Work out the finished part from the listing and answer in its coordinate system (mm). Face numbers are marked on the shaded views. A direction names the side the tool comes from. Round coordinates to 2 decimals unless told otherwise and drop trailing zeros. Order: outer loops, then holes, each group sorted by start corner. A loop starts at its lowest first (then second) coordinate and runs counter-clockwise, first axis right, second up. Notation, with made-up numbers: (35.25, 75.5) - (55.25, 75.5) arc R28 ccw to (55.25, 110.5) - close; hole circle Ø8 at (65.5, -1.75). An arc over 180 degrees is marked (long way). Put each result on its own line as item: value.
Autodesk Inventor part; units mm, degrees
ref_plane "YZ Plane" through (0, 0, 0) normal (1, 0, 0) x (0, 1, 0)
ref_plane "XZ Plane" through (0, 0, 0) normal (0, 1, 0) x (-1, 0, 0)
ref_plane "XY Plane" through (0, 0, 0) normal (0, 0, 1) x (1, 0, 0)
sketch "Sketch1" plane through (0, 0, 0) normal (1, 0, 0) x (0, 1, 0)
  line L0 (0, 0) -> (7.62, 0)
  line L1 (7.62, 0) -> (7.62, -15.24)
  line L2 (7.62, -15.24) -> (0, -15.24)
  line L3 (0, -15.24) -> (0, 0)
  dimension "d0" = 7.62
  dimension "d1" = 15.24
extrude "Extrusion1" add sketch "Sketch1" along normal blind 7.62
ref_plane "Work Plane1" through (0, 3.81, 0) normal (0, 1, 0) x (1, 0, 0)
sketch "Sketch3" plane through (0, 0, 0) normal (-1, 0, 0) x (0, 0, 1)
  line L0 (-2.7422, 2.1047) -> (-12.4487, 2.1047)
  line L1 (-12.4487, 2.1047) -> (-12.4487, 5.5015)
  line L2 (-12.4487, 5.5015) -> (-2.7422, 5.5015)
  line L3 (-2.7422, 5.5015) -> (-2.7422, 2.1047)
  point P0 (0, 0)
extrude "Extrusion2" add sketch "Sketch3" along normal blind 1.27
sketch "Sketch4" plane through (0, 5.5015, -2.7422) normal (0, 1, 0) x (1, 0, 0)
  line L0 (-1.27, 9.7065) -> (-1.27, 0)
  line L1 (-1.27, 0) -> (-52.07, 0)
  line L2 (-52.07, 0) -> (-52.07, 9.7065)
  line L3 (-52.07, 9.7065) -> (-1.27, 9.7065)
  line L4 (-1.27, 9.7065) -> (-1.27, 0)
  point P0 (0, -2.7422)
  dimension "d6" = 50.8
extrude "Extrusion3" add sketch "Sketch4" against normal up to surface (3.3968 mm away)
sketch "Sketch5" plane through (7.62, 0, 0) normal (1, 0, 0) x (0, 0, -1)
  line L0 (15.24, 7.62) -> (15.24, 0)
  line L1 (0, 7.62) -> (15.24, 7.62)
  line L2 (15.24, 0) -> (0, 0)
  line L3 (0, 0) -> (0, 7.62)
  line L4 (0, 7.62) -> (15.24, 7.62)
  line L5 (15.24, 7.62) -> (15.24, 0)
extrude "Extrusion4" cut sketch "Sketch5" against normal blind 3.81
sketch "Sketch6" plane through (0, 7.62, 0) normal (0, 1, 0) x (1, 0, 0)
  line L0 (0, 15.24) -> (3.81, 15.24)
  line L1 (0, 15.24) -> (8.0091, 15.24)
  line L2 (8.0091, 15.24) -> (8.0091, 0)
  line L3 (8.0091, 0) -> (0, 0)
  line L4 (0, 0) -> (0, 15.24)
extrude "Extrusion5" add sketch "Sketch6" along normal blind 1.27
sketch "Sketch7" plane through (0, 0, 0) normal (0, 0, 1) x (1, 0, 0)
  line L0 (3.81, 0) -> (2.54, 0)
  line L1 (2.54, 0) -> (2.54, -7.62)
  line L2 (2.54, -7.62) -> (3.81, -7.62)
  line L3 (3.81, -7.62) -> (3.81, 0)
  point P0 (0, 0)
  dimension "d13" = 1.27
  dimension "d14" = 7.62
extrude "Extrusion6" add sketch "Sketch7" against normal up to surface (15.24 mm away)
fillet "Fillet1" radius 3.175 5 edges at (0, 0, -7.62) (0, 3.8031, -2.7422) (0, 2.1047, -7.5954) (0, 3.8031, -12.4487) (0, 5.5015, -7.5954)
fillet "Fillet2" radius 1 1 edges at (8.0091, 8.89, -7.62)
fillet "Fillet3" radius 1 1 edges at (0, 8.89, -7.62)
properties part number "straightBar"
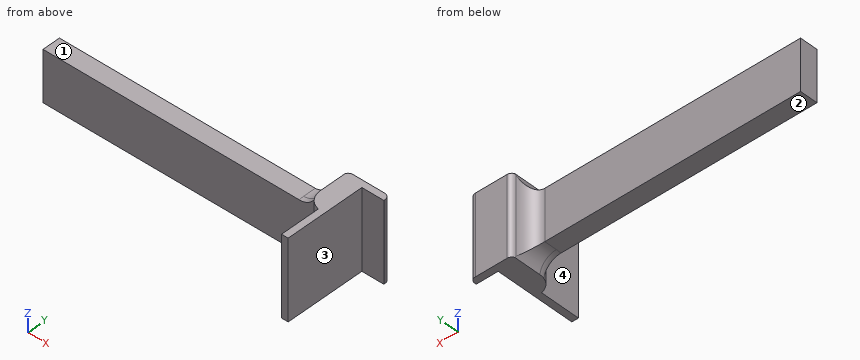
1) Straight lines are drawn through the part: L1, parallel to Z at x = -43, y = 3.5; L2, parallel to Y at x = -26.5, z = -5.75; L3, parallel to X at y = 4.25, z = -3.75. For each, find the intervals that lie inside material, in ascending order. Write a range as from..to.
Findings below:
L1: z = -12.45..-2.74
L2: y = 2.1..5.5
L3: x = -52.07..3.81
2) For the marked faces 1, 2, 3 and 4, determine the directions among +Z, -Z, +X, -X, +Y, -Y from which every point of the face is accessible in a straight line to the end or side of a thin tool.
Findings below:
face 1: +Z, -X, +Y, -Y
face 2: -Z, -X, +Y, -Y
face 3: +Z, -Z, +X, -Y
face 4: +Z, -Z, -X, -Y
3) A cutting plane is placed at D-D on y = -1. Write down the section's boundary in (x, z).
Findings below:
outline: (2.54, -15.24) - (3.81, -15.24) - (3.81, 0) - (2.54, 0) - close
4) A cutting plane is placed at B-B on y = 4.5. Write down the section's boundary in (x, z) (3 decimals).
Findings below:
outline: (-52.07, -12.449) - (-3.152, -12.449) arc R3.175 cw to (0, -15.24) - (3.81, -15.24) - (3.81, 0) - (0, 0) arc R3.175 cw to (-3.145, -2.742) - (-52.07, -2.742) - close
5) Given pin 1 Ø5 at (x, z) = (-27.5, -8) entering from +Y; pin 2 Ø1.5 at (x, z) = (-17.5, -4) entering from -Y; pin 3 Ø1 at (x, y) = (-32.5, 4) entering from -Z, each flat-ended and moving along its own axis, determine where each tip first touches the part or whether it passes through.
Findings below:
pin 1: stops at y = 5.5
pin 2: stops at y = 2.1
pin 3: stops at z = -12.45
6) A cutting plane is placed at C-C on x = -48. Write down the section's boundary in (y, z).
Findings below:
outline: (2.1, -12.45) - (5.5, -12.45) - (5.5, -2.74) - (2.1, -2.74) - close
